Work out the finished part from the listing and answer in its coordinate system (mm). Face numbers are marked on the shaded views. A direction names the side the tool comes from. Coordinates: 2 decimals unless noted, no trailing zeros. Loops run counter-clockwise (first coordinate to the right, second up) from the corner with the lowest first, then second, coordinate; pieces in that order, holes last. Notation, with made-up numbers: (6, 10) - (20, 10) arc R23 cw to (20, 46) - close; hole circle Ø6 at (40.25, 33). An arc over 180 degrees is marked (long way). Write each question's results on one line, items separated by ' | '. Start each with the question number.
Item 1: Section A-A, the plane x = 0 is taken. Write down the section's boundary in (y, z), plus the area to 3 significant figures.
Item 2: Section C-C, the plane y = 27.5 is taken. Write down the section's boundary in (x, z).
Item 3: For a pull along Y with two mould halves and no side action, classify the marked faces 4, 5 and 6 as +Y half, -Y half, draft (parallel to the pull), parting line (faces both ways), or undercut.
Item 4: Each of these flat-tipped pins is pushed along its axis until it touches: pin 1 Ø4.5 at (x, y) = (0, 26) entering from -Z; pin 2 Ø1.5 at (y, z) = (13.5, 0) entering from -X; pin 3 Ø5 at (y, z) = (20.5, 1) entering from -X; pin 4 Ø3 at (y, z) = (3, -2) entering from +X. Where does it stop, or does it pass through?
Item 5: A tool of negligible diameter and unlimited length cuts with its end or side. For the marked faces 1, 2 and 3, from which of +Z, -Z, +X, -X, +Y, -Y can it reach the whole face along a straight path? Write none if from no direction.
Item 6: Consider probe 1 along Z at (x, y) = (3.5, 25); probe 2 along X at (y, z) = (26, -5); probe 3 along X at (y, z) = (-3, 1.25). Determine where each line is inside the solid, lowest interval first. Write a range as [from, to].
Item 7: Section B-B, the plane z = 3.75 is taken. Write down the section's boundary in (x, y), plus the area to 3 significant figures.
Item 8: Section D-D, the plane y = -13 is taken. Write down the section's boundary in (x, z), plus the area to 3 significant figures.
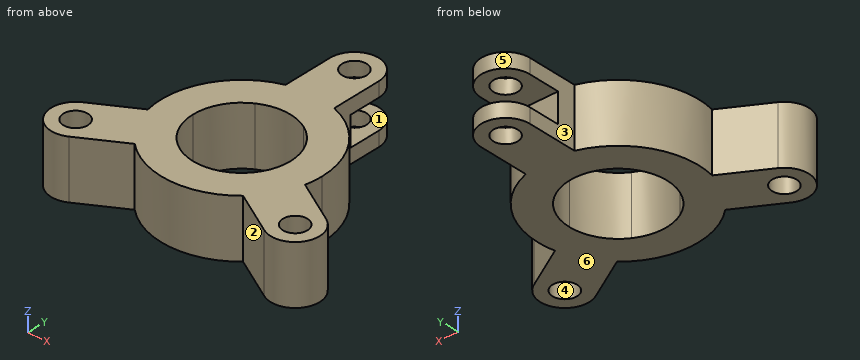
from build123d import *

# Parameters (mm, degrees)
EXTRUDE_1_DEPTH          = 6
EXTRUDE_1_DEPTH_BACK     = 6
SKETCH_1_R               = 2.5
CUT_EXTRUDE_1_DEPTH      = 3
CUT_EXTRUDE_1_DEPTH_BACK = 3
SKETCH_2_W               = 15
SKETCH_2_H               = 13


with BuildPart() as part:
    # Sketch 1 → Extrude 1 (new, two sides: drawn at the far end of the back side and taken through both)
    # profile 1 of 9: a face of its own
    with BuildSketch(Plane.XY.offset(-EXTRUDE_1_DEPTH_BACK)):
        with BuildLine():
            Line((5, 15.724185194), (5, 8.660254038))
            ThreePointArc((5, 8.660254038), (8.660254038, 5), (10, 0))
            Line((10, 0), (16.117543831, -3.531965578))
            ThreePointArc((16.117543831, -3.531965578), (16.404107309, -1.776306108), (16.5, 0))
            ThreePointArc((16.5, 0), (13.318220602, 9.740379869), (5, 15.724185194))
        make_face()
    # profile 2 of 9: a face of its own
    with BuildSketch(Plane.XY.offset(-EXTRUDE_1_DEPTH_BACK)):
        with BuildLine():
            Line((-5, 15.724185194), (-5, 8.660254038))
            ThreePointArc((-5, 8.660254038), (0, 10), (5, 8.660254038))
            Line((5, 8.660254038), (5, 15.724185194))
            ThreePointArc((5, 15.724185194), (0, 16.5), (-5, 15.724185194))
        make_face()
    # profile 3 of 9: a face of its own
    with BuildSketch(Plane.XY.offset(-EXTRUDE_1_DEPTH_BACK)):
        with BuildLine():
            ThreePointArc((-10, 0), (-8.660254038, 5), (-5, 8.660254038))
            Line((-5, 8.660254038), (-5, 15.724185194))
            ThreePointArc((-5, 15.724185194), (-14.289419162, 8.25), (-16.117543831, -3.531965578))
            Line((-16.117543831, -3.531965578), (-10, 0))
        make_face()
    # profile 4 of 9: a face of its own
    with BuildSketch(Plane.XY.offset(-EXTRUDE_1_DEPTH_BACK)):
        with BuildLine():
            ThreePointArc((-5, -8.660254038), (-8.660254038, -5), (-10, 0))
            Line((-10, 0), (-16.117543831, -3.531965578))
            ThreePointArc((-16.117543831, -3.531965578), (-14.289419162, -8.25), (-11.117543831, -12.192219616))
            Line((-11.117543831, -12.192219616), (-5, -8.660254038))
        make_face()
    # profile 5 of 9: a face of its own
    with BuildSketch(Plane.XY.offset(-EXTRUDE_1_DEPTH_BACK)):
        with BuildLine():
            ThreePointArc((5, -8.660254038), (0, -10), (-5, -8.660254038))
            Line((-5, -8.660254038), (-11.117543831, -12.192219616))
            ThreePointArc((-11.117543831, -12.192219616), (0, -16.5), (11.117543831, -12.192219616))
            Line((11.117543831, -12.192219616), (5, -8.660254038))
        make_face()
    # profile 6 of 9: a face of its own
    with BuildSketch(Plane.XY.offset(-EXTRUDE_1_DEPTH_BACK)):
        with BuildLine():
            ThreePointArc((10, 0), (8.660254038, -5), (5, -8.660254038))
            Line((5, -8.660254038), (11.117543831, -12.192219616))
            ThreePointArc((11.117543831, -12.192219616), (14.289419162, -8.25), (16.117543831, -3.531965578))
            Line((16.117543831, -3.531965578), (10, 0))
        make_face()
    # profile 7 of 9: a face of its own
    with BuildSketch(Plane.XY.offset(-EXTRUDE_1_DEPTH_BACK)):
        with BuildLine():
            ThreePointArc((16.117543831, -3.531965578), (14.289419162, -8.25), (11.117543831, -12.192219616))
            Line((11.117543831, -12.192219616), (20.016660498, -17.330127019))
            ThreePointArc((20.016660498, -17.330127019), (26.846787517, -15.5), (25.016660498, -8.669872981))
            Line((25.016660498, -8.669872981), (16.117543831, -3.531965578))
        make_face()
        with Locations((22.516660498, -13)):
            Circle(SKETCH_1_R, mode=Mode.SUBTRACT)
    # profile 8 of 9: a face of its own
    with BuildSketch(Plane.XY.offset(-EXTRUDE_1_DEPTH_BACK)):
        with BuildLine():
            ThreePointArc((-11.117543831, -12.192219616), (-14.289419162, -8.25), (-16.117543831, -3.531965578))
            Line((-16.117543831, -3.531965578), (-25.016660498, -8.669872981))
            ThreePointArc((-25.016660498, -8.669872981), (-26.846787517, -15.5), (-20.016660498, -17.330127019))
            Line((-20.016660498, -17.330127019), (-11.117543831, -12.192219616))
        make_face()
        with Locations((-22.516660498, -13)):
            Circle(SKETCH_1_R, mode=Mode.SUBTRACT)
    # profile 9 of 9: a face of its own
    with BuildSketch(Plane.XY.offset(-EXTRUDE_1_DEPTH_BACK)):
        with BuildLine():
            Line((-5, 26), (-5, 15.724185194))
            ThreePointArc((-5, 15.724185194), (0, 16.5), (5, 15.724185194))
            Line((5, 15.724185194), (5, 26))
            ThreePointArc((5, 26), (0, 31), (-5, 26))
        make_face()
        with Locations((0, 26)):
            Circle(SKETCH_1_R, mode=Mode.SUBTRACT)
    extrude(amount=EXTRUDE_1_DEPTH + EXTRUDE_1_DEPTH_BACK)

    # Sketch 2 → Cut-Extrude 1 (cut, two sides: drawn at the far end of the back side and taken through both)
    with BuildSketch(Plane.XY.offset(-CUT_EXTRUDE_1_DEPTH_BACK)):
        with Locations((0, 26)):
            Rectangle(SKETCH_2_W, SKETCH_2_H)
    extrude(amount=CUT_EXTRUDE_1_DEPTH + CUT_EXTRUDE_1_DEPTH_BACK, mode=Mode.SUBTRACT)


solid = part.part
Answer key:
1) outline: (-16.5, -6) - (-10, -6) - (-10, 6) - (-16.5, 6) - close; (10, -6) - (23.5, -6) - (23.5, -3) - (19.5, -3) - (19.5, 3) - (23.5, 3) - (23.5, 6) - (10, 6) - close; (28.5, -6) - (31, -6) - (31, -3) - (28.5, -3) - close; (28.5, 3) - (31, 3) - (31, 6) - (28.5, 6) - close | area: 231 mm^2
2) outline: (-4.77, -6) - (-2, -6) - (-2, -3) - (-4.77, -3) - close; (-4.77, 3) - (-2, 3) - (-2, 6) - (-4.77, 6) - close; (2, -6) - (4.77, -6) - (4.77, -3) - (2, -3) - close; (2, 3) - (4.77, 3) - (4.77, 6) - (2, 6) - close
3) face 4: undercut | face 5: +Y half | face 6: draft
4) pin 1: passes through | pin 2: stops at x = -10.47 | pin 3: stops at x = -5 | pin 4: stops at x = 16.43
5) face 1: +X, -X, +Y | face 2: +Z, -Z, -Y | face 3: +Z, -Z, -X, +Y
6) probe 1: z = [-6, -3], [3, 6] | probe 2: x = [-5, -2.5], [2.5, 5] | probe 3: x = [-16.22, -9.54], [9.54, 16.22]
7) outline: (-25.02, -8.67) arc R5 ccw to (-20.02, -17.33) - (-11.12, -12.19) arc R16.5 ccw to (11.12, -12.19) - (20.02, -17.33) arc R5 ccw to (25.02, -8.67) - (16.12, -3.53) arc R16.5 ccw to (5, 15.72) - (5, 26) arc R5 ccw to (-5, 26) - (-5, 15.72) arc R16.5 ccw to (-16.12, -3.53) - close; hole circle Ø5 at (-22.52, -13); hole circle Ø20 at (0, 0); hole circle Ø5 at (0, 26); hole circle Ø5 at (22.52, -13) | area: 893 mm^2
8) outline: (-27.52, -6) - (-25.02, -6) - (-25.02, 6) - (-27.52, 6) - close; (-20.02, -6) - (-12.52, -6) - (-12.52, 6) - (-20.02, 6) - close; (-10.16, -6) - (10.16, -6) - (10.16, 6) - (-10.16, 6) - close; (12.52, -6) - (20.02, -6) - (20.02, 6) - (12.52, 6) - close; (25.02, -6) - (27.52, -6) - (27.52, 6) - (25.02, 6) - close | area: 484 mm^2
